Autodesk Inventor part; units mm, degrees
ref_plane "YZ Plane" through (0, 0, 0) normal (1, 0, 0) x (0, 1, 0)
ref_plane "XZ Plane" through (0, 0, 0) normal (0, 1, 0) x (-1, 0, 0)
ref_plane "XY Plane" through (0, 0, 0) normal (0, 0, 1) x (1, 0, 0)
sketch "Sketch1" plane through (0, 0, 0) normal (0, 1, 0) x (-1, 0, 0)
  line L0 (0, 0) -> (-25, 0)
  line L1 (-25, 0) -> (-25, -25)
  line L2 (-25, -25) -> (0, -25)
  line L3 (0, -25) -> (0, 0)
  line L4 (-23.5, -23.5) -> (-23.5, -1.5)
  line L5 (-23.5, -1.5) -> (-1.5, -1.5)
  line L6 (-1.5, -1.5) -> (-1.5, -23.5)
  line L7 (-1.5, -23.5) -> (-23.5, -23.5)
  dimension "d0" = 25
  dimension "d1" = 25
  dimension "d2" = 1.5
extrude "Extrusion1" add sketch "Sketch1" along normal blind 100
sketch "Sketch2" plane through (25, 0, 0) normal (1, 0, 0) x (0, 0, -1)
  line L0 (0, 100) -> (25, 100)
  point P0 (0, 0)
  point P1 (12.5, 85)
  point P2 (12.5, 65)
  point P3 (12.5, 12.5)
  dimension "d5" = 35
  dimension "d6" = 15
  dimension "d7" = 12.5
  dimension "d15" = 12.5
hole "Hole1" at (25, 85, -12.5) at (25, 65, -12.5) at (25, 12.5, -12.5) direction (-1, 0, 0) diameter 6 end through all
sketch "Sketch3" plane through (25, 0, -25) normal (0, 0, -1) x (-1, 0, 0)
  line L0 (0, 100) -> (25, 100)
  point P0 (25, 0)
  point P1 (12.5, 75)
  dimension "d16" = 25
  dimension "d17" = 12.5
hole "Hole2" at (12.5, 75, -25) direction (0, 0, 1) diameter 6 end through all
properties part number "Side Bar Mount"
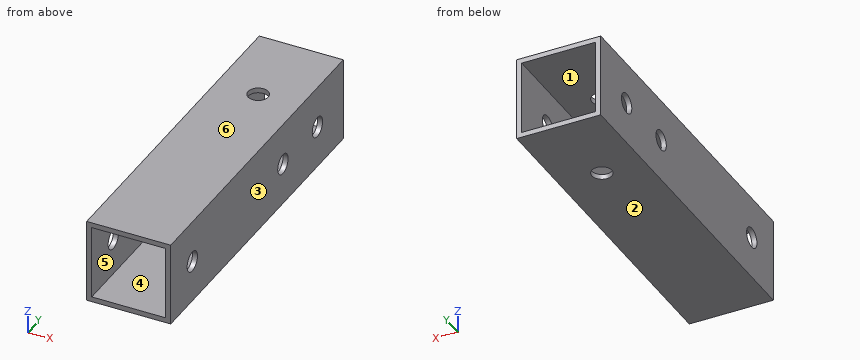
CAD build for the part. Positions are in the model's coordinates, mm. Face numbers are marked on the shaded views. A direction names the side the tool comes from. Round coordinates to 2 decimals unless told otherwise and drop trailing zeros. Order: outer loops, then holes, each group sorted by start corner. A loop starts at its lowest first (then second) coordinate and runs counter-clockwise, first axis right, second up.
Q1. Wall check: L1, parallel to Y at x = 0.85, z = -12.5; L2, parallel to X at y = 22, z = -15; L3, parallel to Z at x = 0.85, y = 65. Give the ranges that are in metal, low to high.
Q2. Two-plate mould, pull along X, no slides. Class the marked faces 1, 2, 3 and 4: pulls with the +X half, pulls with the -X half, needs draft (parallel to the pull), parting line crosses it, or undercut.
Q3. Which spindle directions (+Z, -Z, +X, -X, +Y, -Y) get a long thin tool onto all of the face, cutting with end or side? Do the marked faces 5 and 6. Say none if no direction does.
Q4. Slice it at B-B (y = 65). Write the cut outline in (x, z).
Q5. Slice it at D-D (z = -12.5). State how many separate pieces and enclosed holes the cut face has, and give its area (3 significant figures).
Q6. Slice it at C-C (x = 5.25). Write the cut outline in (y, z).
Q7. Drop a flat-ended pin along its axis: pin 1 (8 mm diameter, centred on x = 12.5, y = 75, fed in from +Z). Give the stop position or say it passes through.
Q8. Slice it at A-A (z = -7.25). Write the cut outline in (x, y), and give its area (3 significant figures).
Results below:
1. L1: y = 0 to 9.5, 15.5 to 62, 68 to 82, 88 to 100
1. L2: x = 0 to 1.5, 23.5 to 25
1. L3: z = -25 to -15.5, -9.5 to 0
2. face 1: undercut
2. face 2: needs draft
2. face 3: pulls with the +X half
2. face 4: undercut
3. face 5: +Y, -Y
3. face 6: +Z, +X, -X, +Y, -Y
4. outline: (0, -25) - (25, -25) - (25, -15.5) - (23.5, -15.5) - (23.5, -23.5) - (1.5, -23.5) - (1.5, -15.5) - (0, -15.5) - close; (0, -9.5) - (1.5, -9.5) - (1.5, -1.5) - (23.5, -1.5) - (23.5, -9.5) - (25, -9.5) - (25, 0) - (0, 0) - close
5. separate pieces: 8
5. enclosed holes: 0
5. area: 246 mm2
6. outline: (0, -25) - (100, -25) - (100, -23.5) - (0, -23.5) - close; (0, -1.5) - (100, -1.5) - (100, 0) - (0, 0) - close
7. pin 1: stops at z = 0
8. outline: (0, 0) - (1.5, 0) - (1.5, 100) - (0, 100) - close; (23.5, 0) - (25, 0) - (25, 100) - (23.5, 100) - close
8. area: 300 mm2
